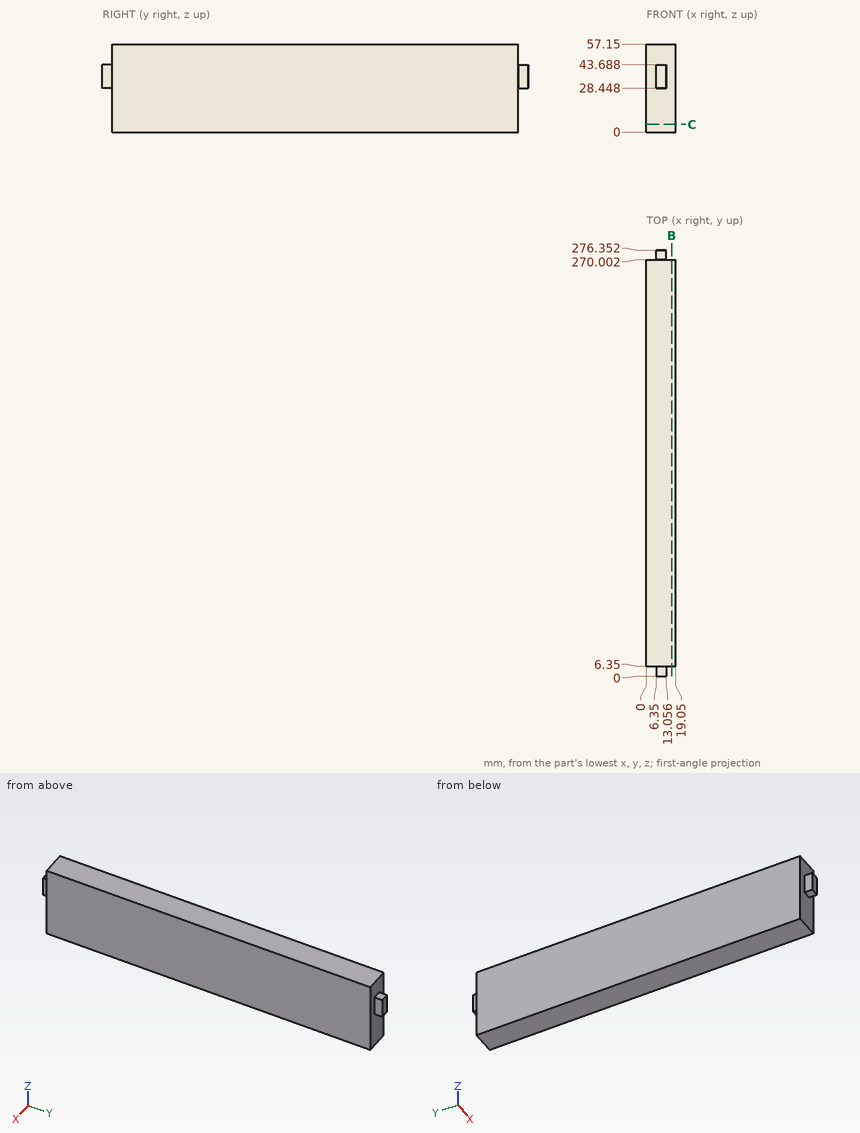
Source: three-view drawing plus pictorial views. Frame: mm from the lowest corner of the part. Round coordinates to 2 decimals unless told otherwise and drop trailing zeros. Loops run counter-clockwise (first coordinate to the right, second up) from the corner with the lowest first, then second, coordinate; pieces in that order, holes last.
Q1. Section C-C on z = 5. Return loops of the section in (x, y), plus the area to 3 significant figures.
Q2. Material intervals for L1, parallel to Y at x = 4.5, z = 11.5, sorted ascending.
Q3. Section B-B on x = 16.5. Return loops of the section in (y, z).
Q4. Pin query (flat end, axial travel): P1, Ø5, axis at y = 4.5, z = 36, coming from the +X side; P2, Ø5, axis at x = 17, z = 29, coming from the -Y side; P3, Ø1.9, axis at y = 273.5, z = 33, coming from the +X side; P4, Ø5, axis at x = 8.5, y = 3, coming from the +Z side. Return the tip coordinate at first contact, or that it passes through.
Evaluation:
1. outline: (0, 6.35) - (19.05, 6.35) - (19.05, 270) - (0, 270) - close
1. area: 5,020 mm2
2. L1: y = 6.35 to 270
3. outline: (6.35, 0) - (270, 0) - (270, 57.15) - (6.35, 57.15) - close
4. P1: stops at x = 19.05
4. P2: stops at y = 6.35
4. P3: stops at x = 13.06
4. P4: stops at z = 43.69
